Model file for the job. Use its own axes, mm. Coordinates: 2 decimals unless noted, no trailing zeros. Order: outer loops, then holes, each group sorted by start corner. A loop starts at its lowest first (then second) coordinate and runs counter-clockwise, first axis right, second up. Notation, with made-up numbers: M 11.5,-25.5 L 52.5,-25.5 A24 cw 52.5,7.5 Z; hole C -32.5,77 d10. An arc over 180 degrees is marked long. Return JSON: item names as keys, results as strings.
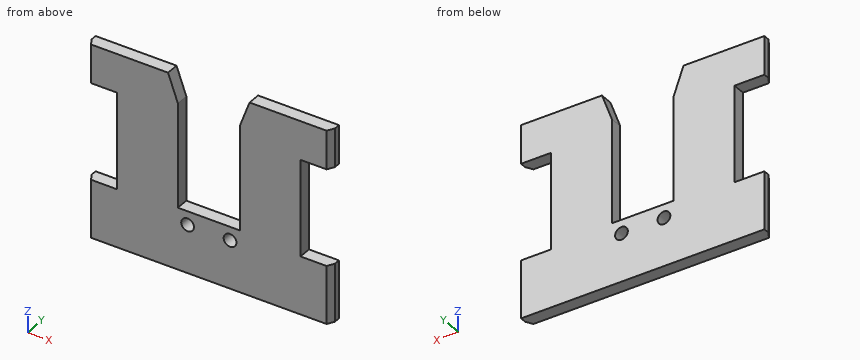
```python
from build123d import *

# Parameters (mm, degrees)
F0_R     = 1.651
F1_DEPTH = 1.651
F2_SIZE2 = 1.7597636205
F2_SIZE  = 1.016


with BuildPart() as f1:
    # F0 (on Front) → F1 (new body, symmetric)
    with BuildSketch(Plane.XZ):
        Polygon((-31.5087, -7.5057), (31.5087, -7.5057), (31.5087, 7.5057), (23.7617, 7.5057), (23.7617, 32.4993), (31.5087, 32.4993), (31.5087, 42.5069), (23.7617, 42.5069), (10.5537, 42.5069), (8.0137, 35.4965), (8.0137, 8.4963), (0, 8.4963), (-8.0137, 8.4963), (-8.0137, 35.4965), (-10.5537, 42.5069), (-23.7617, 42.5069), (-31.5087, 42.5069), (-31.5087, 32.4993), (-23.7617, 32.4993), (-23.7617, 7.5057), (-31.5087, 7.5057), align=None)
        with Locations((-5.4991, 4.9910574029)):
            Circle(F0_R, mode=Mode.SUBTRACT)
        with Locations((5.4991, 4.9910574029)):
            Circle(F0_R, mode=Mode.SUBTRACT)
    extrude(amount=F1_DEPTH, both=True)

    # F2
    f2_edges = [f1.edges().sort_by_distance(p)[0] for p in [
        (31.5087, -1.651, 0),
        (31.5087, -1.651, 37.5031),
        (-31.5087, -1.651, 0),
        (-31.5087, -1.651, 37.5031),
    ]]
    f2_side = f1.faces().sort_by_distance((0, -1.651, -6.701184))[0]
    chamfer(f2_edges, length=F2_SIZE, length2=F2_SIZE2, reference=f2_side)


solid = f1.part
```
Item 1: Saw through at B-B (z = 23). Write the cut outline in (x, y).
Check result:
{"outline": "M -23.76,-1.65 L -8.01,-1.65 L -8.01,1.65 L -23.76,1.65 Z; M 8.01,-1.65 L 23.76,-1.65 L 23.76,1.65 L 8.01,1.65 Z"}
Item 2: Wall check: line 1 (Z direction, x = -27, y = -1.4); line 2 (X direction, y = -0.35, z = 12); line 3 (Z direction, x = 5.5, y = -0.85). Give the ranges that are in metal, low to high.
Check result:
{"line 1": "z = -7.51 to 7.51, 32.5 to 42.51", "line 2": "x = -23.76 to -8.01, 8.01 to 23.76", "line 3": "z = -7.51 to 3.34, 6.64 to 8.5"}
Item 3: Drop flat-ended pins along their axis: pin 1 Ø1 at (y, z) = (0.5, 16.5) entering from -X; pin 2 Ø1.5 at (y, z) = (-0.5, 11.5) entering from +X; pin 3 Ø1 at (x, y) = (1.5, -0.5) entering from +Z; pin 4 Ø5.5 at (x, z) = (-5.5, 4.99) entering from +Y. Give the stop position or say it passes through.
Check result:
{"pin 1": "stops at x = -23.76", "pin 2": "stops at x = 23.76", "pin 3": "stops at z = 8.5", "pin 4": "stops at y = 1.65"}
Item 4: Saw through at C-C (x = -1). Write the cut outline in (y, z).
Check result:
{"outline": "M -1.65,-7.51 L 1.65,-7.51 L 1.65,8.5 L -1.65,8.5 Z"}
Item 5: Saw through at A-A (x = 5.5). Write the cut outline in (y, z), and give its area (3 significant figures).
Check result:
{"outline": "M -1.65,-7.51 L 1.65,-7.51 L 1.65,3.34 L -1.65,3.34 Z; M -1.65,6.64 L 1.65,6.64 L 1.65,8.5 L -1.65,8.5 Z", "area": "41.9 mm2"}
